CAD build for the part. Positions are in the model's coordinates, mm. A direction names the side the tool comes from. Give positions to 0.01 mm unless a question says otherwise; leave off trailing zeros. Order: outer loops, then holes, each group sorted by start corner. A loop starts at its lowest first (then second) coordinate and runs counter-clockwise, first axis right, second up. Notation, with made-up numbers: M 76,-30.5 L 89,-30.5 A18 cw 89,-9.5 Z; hole C -35.5,56 d5. An arc over 180 degrees is marked long. Put each result on its own line as item: value. Start each with the question number.
1) Tool access for faces 4 (the face through (19.268, 46.138, 9.86)), 5 (the face through (48.03, -37.12, 9.86)), 6 (the face through (-2.17, -9.76, -14.79)): list every direction of +Z, -Z, +X, -X, +Y, -Y with a clear straight run to the whole face (end or side of a thin tool).
2) Cut at A-A (x = 0). Write the cut outline in (y, z), and give its area (3 significant figures).
3) Two-plate mould, pull along Y, no slides. Class faces 1 (the face through (47.884, 36.848, 9.86)), 2 (the face through (19, -46.25, 9.86)), 3 (the face through (37.12, 48.03, 9.86)): released by +Y, released by -Y, zero draft, split by the parting line, or undercut.
4) Cut at C-C (z = 74.5). Write the cut outline in (x, y), and give its area (3 significant figures).
5) Cut at D-D (y = -45). Write the cut outline in (x, z), and give its area (3 significant figures).
6) Pin check, flat tips, straight feed: pin 1 (12 mm diameter, centred on x = 36.5, y = -22, fed in from +Z); pin 2 (8 mm diameter, centred on x = 0, y = 0, fed in from -Z); pin 3 (1.5 mm diameter, centred on y = 19.5, z = 7, fed in from +X); pin 4 (1.5 mm diameter, centred on x = -45, y = -47.5, fed in from -Z). Stop position of each tip, or through.
7) Drill centre lines: line 1 (Y direction, x = 0, z = 80); line 2 (Z direction, x = 29, y = -31.5); line 3 (Y direction, x = 0, z = 13). Where is each one in solid material? Low to high. Write a range as [from, to].
```python
from build123d import *

# Parameters (mm, degrees)
F1_DEPTH      = 20
F2_R          = 10
F3_DEPTH      = 120
F3_DEPTH_BACK = 50
F4_R          = 5
F5_DEPTH      = 170


with BuildPart() as f1:
    # F0 (on Top) → F1 (new body)
    with BuildSketch(Plane.XY):
        with BuildLine():
            ThreePointArc((49.143051, -9.217405), (49.785302, -4.628578), (50, 0))
            ThreePointArc((50, 0), (49.785302, 4.628578), (49.143051, 9.217405))
            ThreePointArc((49.143051, 9.217405), (46.193977, 19.134172), (41.267074, 28.231695))
            ThreePointArc((41.267074, 28.231695), (35.355339, 35.355339), (28.231695, 41.267074))
            ThreePointArc((28.231695, 41.267074), (19.134172, 46.193977), (9.217405, 49.143051))
            ThreePointArc((9.217405, 49.143051), (4.628578, 49.785302), (0, 50))
            ThreePointArc((0, 50), (-4.628578, 49.785302), (-9.217405, 49.143051))
            ThreePointArc((-9.217405, 49.143051), (-19.134172, 46.193977), (-28.231695, 41.267074))
            ThreePointArc((-28.231695, 41.267074), (-35.355339, 35.355339), (-41.267074, 28.231695))
            ThreePointArc((-41.267074, 28.231695), (-46.193977, 19.134172), (-49.143051, 9.217405))
            ThreePointArc((-49.143051, 9.217405), (-50, 0), (-49.143051, -9.217405))
            ThreePointArc((-49.143051, -9.217405), (-46.193977, -19.134172), (-41.267074, -28.231695))
            ThreePointArc((-41.267074, -28.231695), (-35.355339, -35.355339), (-28.231695, -41.267074))
            ThreePointArc((-28.231695, -41.267074), (-19.134172, -46.193977), (-9.217405, -49.143051))
            ThreePointArc((-9.217405, -49.143051), (0, -50), (9.217405, -49.143051))
            ThreePointArc((9.217405, -49.143051), (19.134172, -46.193977), (28.231695, -41.267074))
            ThreePointArc((28.231695, -41.267074), (35.355339, -35.355339), (41.267074, -28.231695))
            ThreePointArc((41.267074, -28.231695), (46.193977, -19.134172), (49.143051, -9.217405))
        make_face()
        with BuildLine():
            ThreePointArc((49.143051, 9.217405), (49.785302, 4.628578), (50, 0))
            ThreePointArc((50, 0), (49.785302, -4.628578), (49.143051, -9.217405))
            ThreePointArc((49.143051, -9.217405), (60.063704, -7.759767), (70, -3))
            Line((70, -3), (70, 0))
            Line((70, 0), (70, 3))
            ThreePointArc((70, 3), (60.063704, 7.759767), (49.143051, 9.217405))
        make_face()
        with BuildLine():
            ThreePointArc((28.231695, 41.267074), (35.355339, 35.355339), (41.267074, 28.231695))
            ThreePointArc((41.267074, 28.231695), (47.958436, 36.984468), (51.618795, 47.376154))
            Line((51.618795, 47.376154), (49.497475, 49.497475))
            Line((49.497475, 49.497475), (47.376154, 51.618795))
            ThreePointArc((47.376154, 51.618795), (36.984468, 47.958436), (28.231695, 41.267074))
        make_face()
        with BuildLine():
            ThreePointArc((51.618795, -47.376154), (47.958436, -36.984468), (41.267074, -28.231695))
            ThreePointArc((41.267074, -28.231695), (35.355339, -35.355339), (28.231695, -41.267074))
            ThreePointArc((28.231695, -41.267074), (36.984468, -47.958436), (47.376154, -51.618795))
            Line((47.376154, -51.618795), (49.497475, -49.497475))
            Line((49.497475, -49.497475), (51.618795, -47.376154))
        make_face()
        with BuildLine():
            ThreePointArc((0, 50), (4.628578, 49.785302), (9.217405, 49.143051))
            ThreePointArc((9.217405, 49.143051), (7.759767, 60.063704), (3, 70))
            Line((3, 70), (0, 70))
            Line((0, 70), (0, 50))
        make_face()
        with BuildLine():
            ThreePointArc((3, -70), (7.759767, -60.063704), (9.217405, -49.143051))
            ThreePointArc((9.217405, -49.143051), (0, -50), (-9.217405, -49.143051))
            ThreePointArc((-9.217405, -49.143051), (-7.759767, -60.063704), (-3, -70))
            Line((-3, -70), (0, -70))
            Line((0, -70), (3, -70))
        make_face()
        with BuildLine():
            ThreePointArc((-9.217405, 49.143051), (-4.628578, 49.785302), (0, 50))
            Line((0, 50), (0, 70))
            Line((0, 70), (-3, 70))
            ThreePointArc((-3, 70), (-7.759767, 60.063704), (-9.217405, 49.143051))
        make_face()
        with BuildLine():
            ThreePointArc((-47.376154, -51.618795), (-36.984468, -47.958436), (-28.231695, -41.267074))
            ThreePointArc((-28.231695, -41.267074), (-35.355339, -35.355339), (-41.267074, -28.231695))
            ThreePointArc((-41.267074, -28.231695), (-47.958436, -36.984468), (-51.618795, -47.376154))
            Line((-51.618795, -47.376154), (-49.497475, -49.497475))
            Line((-49.497475, -49.497475), (-47.376154, -51.618795))
        make_face()
        with BuildLine():
            ThreePointArc((-41.267074, 28.231695), (-35.355339, 35.355339), (-28.231695, 41.267074))
            ThreePointArc((-28.231695, 41.267074), (-36.984468, 47.958436), (-47.376154, 51.618795))
            Line((-47.376154, 51.618795), (-49.497475, 49.497475))
            Line((-49.497475, 49.497475), (-51.618795, 47.376154))
            ThreePointArc((-51.618795, 47.376154), (-47.958436, 36.984468), (-41.267074, 28.231695))
        make_face()
        with BuildLine():
            ThreePointArc((-70, -3), (-60.063704, -7.759767), (-49.143051, -9.217405))
            ThreePointArc((-49.143051, -9.217405), (-50, 0), (-49.143051, 9.217405))
            ThreePointArc((-49.143051, 9.217405), (-60.063704, 7.759767), (-70, 3))
            Line((-70, 3), (-70, 0))
            Line((-70, 0), (-70, -3))
        make_face()
    extrude(amount=F1_DEPTH)

    # F2 (on face) → F3 (join, two sides)
    with BuildSketch(Plane.XY.offset(20)) as f3_sk:
        Circle(F2_R)
    extrude(amount=F3_DEPTH)
    extrude(f3_sk.sketch, amount=-F3_DEPTH_BACK)

    # F4 (on face) → F5 (cut, through all)
    with BuildSketch(Plane.XY.offset(140)):
        Circle(F4_R)
    extrude(amount=-F5_DEPTH, mode=Mode.SUBTRACT)


solid = f1.part
```
Solution:
1. face 4: +Z, -Z, +Y
1. face 5: +Z, -Z, +X
1. face 6: -Z
2. outline: M -70,0 L -10,0 L -10,-30 L -5,-30 L -5,140 L -10,140 L -10,20 L -70,20 Z; M 5,-30 L 10,-30 L 10,0 L 70,0 L 70,20 L 10,20 L 10,140 L 5,140 Z
2. area: 4,100 mm²
3. face 1: undercut
3. face 2: released by -Y
3. face 3: released by +Y
4. outline: C 0,0 d20; hole C 0,0 d10
4. area: 236 mm²
5. outline: M -51.1,0 L -32.4,0 L -32.4,20 L -51.1,20 Z; M -21.79,0 L 21.79,0 L 21.79,20 L -21.79,20 Z; M 32.4,0 L 51.1,0 L 51.1,20 L 32.4,20 Z
5. area: 1,620 mm²
6. pin 1: z = 20
6. pin 2: through
6. pin 3: x = 46.35
6. pin 4: z = 0
7. line 1: [-10, -5], [5, 10]
7. line 2: [0, 20]
7. line 3: [-70, -5], [5, 70]
